Design review of the part built by this model. Coordinates are the model's own, in mm. Face numbers are marked on the shaded views. Coordinates: 2 decimals unless noted, no trailing zeros. Loops run counter-clockwise (first coordinate to the right, second up) from the corner with the lowest first, then second, coordinate; pieces in that order, holes last. Notation, with made-up numbers: (9.25, -10) - (65.25, -10) arc R31 ccw to (65.25, 14) - close; hole circle Ø9 at (-4, 34). An arc over 180 degrees is marked (long way). Answer in a Markdown table with one row per item. Add a question column.
(1) We need section D-D, the plane y = 13. Write out the cut boundary in (x, z).
(2) We need section A-A, the plane z = 31. Write out the cut boundary in (x, y).
(3) Clearance check with flat-ended pins moving along their axes: pin 1 (1.8 mm diameter, centred on x = 4.5, y = 53.5, fed in from +Z); pin 2 (2.5 mm diameter, centred on x = 4.5, y = 4.5, fed in from -Z); pin 3 (1.8 mm diameter, centred on x = 152, y = 52, fed in from +Z). State where each tip first meets the part, or that it passes through.
(4) To check wall thickness, follow L1, parallel to Y at x = 152.5, z = 36.75; L2, parallel to Y at x = 99.5, z = 30; L3, parallel to X at y = 41, z = 22.5. State the ranges of each line that lie inside material, in increasing order. Write a range as [from, to].
(5) We need section C-C, the plane z = 18.5. Write out the cut boundary in (x, y).
(6) The part is to be moulded in two halves that separate along Y. For the marked faces 1, 2, 3 and 4, say which applies: released by +Y, released by -Y, zero draft, split by the parting line, or undercut.
(7) We need section B-B, the plane y = 31. Write out the cut boundary in (x, z).
from build123d import *

# Parameters (mm, degrees)
SKETCH_W        = 157
SKETCH_H        = 58
PAD_DEPTH       = 1
SKETCH001_W     = 157
SKETCH001_H     = 58
SKETCH001_W_2   = 154
SKETCH001_H_2   = 55
PAD001_DEPTH    = 50
SKETCH002_W     = 6
SKETCH002_H     = 6
PAD002_DEPTH    = 47
SKETCH003_R     = 1
POCKET_DEPTH    = 20
SKETCH004_W     = 4
SKETCH004_H     = 10
SKETCH004_W_2   = 8.1
SKETCH004_H_2   = 8.1
PAD003_DEPTH    = 5
SKETCH005_R     = 1
POCKET001_DEPTH = 5
SKETCH006_W     = 10
SKETCH006_H     = 5
POCKET002_DEPTH = 1.5
FILLET_R        = 1


with BuildPart() as part:
    # Sketch → Pad (new body)
    with BuildSketch(Plane.XY):
        with Locations((78.5, 29)):
            Rectangle(SKETCH_W, SKETCH_H)
    extrude(amount=PAD_DEPTH)

    # Sketch001 (on Face6 of Pad) → Pad001 (join)
    with BuildSketch(Plane.XY.offset(1)):
        with Locations((78.5, 29)):
            Rectangle(SKETCH001_W, SKETCH001_H)
        with Locations((78.5, 29)):
            Rectangle(SKETCH001_W_2, SKETCH001_H_2, mode=Mode.SUBTRACT)
    extrude(amount=PAD001_DEPTH)

    # Sketch002 (on Face15 of Pad001) → Pad002 (join)
    with BuildSketch(Plane.XY.offset(1)):
        with Locations((4.5, 53.5)):
            Rectangle(SKETCH002_W, SKETCH002_H)
        with Locations((152.5, 53.5)):
            Rectangle(SKETCH002_W, SKETCH002_H)
        with Locations((152.5, 4.5)):
            Rectangle(SKETCH002_W, SKETCH002_H)
        with Locations((4.5, 4.5)):
            Rectangle(SKETCH002_W, SKETCH002_H)
    extrude(amount=PAD002_DEPTH)

    # Sketch003 (on Face15 of Pad002) → Pocket (cut)
    with BuildSketch(Plane.XY.offset(48)):
        with Locations((4.5, 53.5)):
            Circle(SKETCH003_R)
        with Locations((4.5, 4.5)):
            Circle(SKETCH003_R)
        with Locations((152.5, 4.5)):
            Circle(SKETCH003_R)
        with Locations((152.5, 53.5)):
            Circle(SKETCH003_R)
    extrude(amount=-POCKET_DEPTH, mode=Mode.SUBTRACT)

    # Sketch004 (on Face17 of Pocket) → Pad003 (join)
    with BuildSketch(Plane.XY.offset(1)):
        with Locations((3.5, 38.05)):
            Rectangle(SKETCH004_W, SKETCH004_H)
        with Locations((3.5, 19.95)):
            Rectangle(SKETCH004_W, SKETCH004_H)
        with Locations((49.55, 29)):
            Rectangle(SKETCH004_W_2, SKETCH004_H_2)
    extrude(amount=PAD003_DEPTH)

    # Sketch005 (on Face28 of Pad003) → Pocket001 (cut)
    with BuildSketch(Plane.XY.offset(6)):
        with Locations((3.5, 34.7)):
            Circle(SKETCH005_R)
        with Locations((3.5, 23.3)):
            Circle(SKETCH005_R)
    extrude(amount=-POCKET001_DEPTH, mode=Mode.SUBTRACT)

    # Sketch006 (on Face7 of Pocket001) → Pocket002 (cut)
    with BuildSketch(Plane(origin=(0, 0, 0), x_dir=(0, -1, 0), z_dir=(-1, 0, 0))):
        with Locations((-29, 8.5)):
            Rectangle(SKETCH006_W, SKETCH006_H)
    extrude(amount=-POCKET002_DEPTH, mode=Mode.SUBTRACT)

    # Fillet
    fillet_edges = [part.edges().sort_by_distance(p)[0] for p in [
        (157, 0, 26),
        (157, 58, 26),
        (0, 58, 26),
        (0, 0, 26),
    ]]
    fillet(fillet_edges, radius=FILLET_R)


solid = part.part
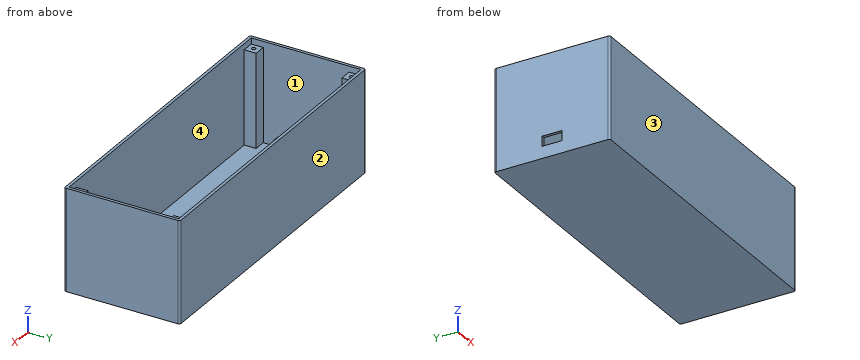
Responses:
| question | item | result |
|---|---|---|
| 1 | outline | (0, 0) - (157, 0) - (157, 51) - (155.5, 51) - (155.5, 1) - (1.5, 1) - (1.5, 51) - (0, 51) - close |
| 2 | outline | (0, 1) arc R1 ccw to (1, 0) - (156, 0) arc R1 ccw to (157, 1) - (157, 57) arc R1 ccw to (156, 58) - (1, 58) arc R1 ccw to (0, 57) - close; hole (1.5, 7.5) - (7.5, 7.5) - (7.5, 1.5) - (149.5, 1.5) - (149.5, 7.5) - (155.5, 7.5) - (155.5, 50.5) - (149.5, 50.5) - (149.5, 56.5) - (7.5, 56.5) - (7.5, 50.5) - (1.5, 50.5) - close; hole circle Ø2 at (4.5, 4.5); hole circle Ø2 at (4.5, 53.5); hole circle Ø2 at (152.5, 4.5); hole circle Ø2 at (152.5, 53.5) |
| 3 | pin 1 | stops at z = 28 |
| 3 | pin 2 | stops at z = 0 |
| 3 | pin 3 | stops at z = 48 |
| 4 | L1 | y = [0, 3.5], [5.5, 7.5], [50.5, 52.5], [54.5, 58] |
| 4 | L2 | y = [0, 1.5], [56.5, 58] |
| 4 | L3 | x = [0, 1.5], [155.5, 157] |
| 5 | outline | (0, 1) arc R1 ccw to (1, 0) - (156, 0) arc R1 ccw to (157, 1) - (157, 57) arc R1 ccw to (156, 58) - (1, 58) arc R1 ccw to (0, 57) - close; hole (1.5, 7.5) - (7.5, 7.5) - (7.5, 1.5) - (149.5, 1.5) - (149.5, 7.5) - (155.5, 7.5) - (155.5, 50.5) - (149.5, 50.5) - (149.5, 56.5) - (7.5, 56.5) - (7.5, 50.5) - (1.5, 50.5) - close |
| 6 | face 1 | undercut |
| 6 | face 2 | released by +Y |
| 6 | face 3 | released by -Y |
| 6 | face 4 | undercut |
| 7 | outline | (0, 0) - (157, 0) - (157, 51) - (155.5, 51) - (155.5, 1) - (53.6, 1) - (53.6, 6) - (45.5, 6) - (45.5, 1) - (1.5, 1) - (1.5, 6) - (0, 6) - close; (0, 11) - (1.5, 11) - (1.5, 51) - (0, 51) - close |
